Input: part model. Units: mm. Frame: model coordinates. A direction names the side the tool comes from. Coordinates: 2 decimals unless noted, no trailing zeros. Order: outer loops, then holes, each group sorted by start corner. A loop starts at its lowest first (then second) coordinate and runs counter-clockwise, first axis right, second up.
from build123d import *

# Parameters (mm, degrees)
MODEL_R                 = 6
MODEL_W                 = 3
MODEL_H                 = 24
SALIENTE_EXTRUIR2_DEPTH = 3


with BuildPart() as part:
    # Model → Saliente-Extruir2 (new body)
    with BuildSketch(Plane.XY):
        Polygon((-39.51128192, -9.185059482), (-32.41128192, -9.185059482), (-32.41128192, 2.614940518), (-9.21128192, 2.614940518), (-9.21128192, -9.185059482), (16.002025332, -9.185059482), (50.517196398, -9.185059482), (78.48871808, -9.185059482), (89.48871808, -9.185059482), (96.48871808, -9.185059482), (103.48871808, -9.185059482), (108.48871808, -9.185059482), (108.48871808, 88.814940518), (24.48871808, 88.814940518), (2.28871808, 88.814940518), (-0.51128192, 88.814940518), (-1.51128192, 88.814940518), (-9.21128192, 88.814940518), (-9.21128192, 77.014940518), (-32.41128192, 77.014940518), (-32.41128192, 88.814940518), (-39.51128192, 88.814940518), align=None)
        with Locations((-12.040844912, 39.714244751)):
            Circle(MODEL_R, mode=Mode.SUBTRACT)
        with Locations((-31.01128192, 39.814940518)):
            Rectangle(MODEL_W, MODEL_H, mode=Mode.SUBTRACT)
    extrude(amount=SALIENTE_EXTRUIR2_DEPTH)


solid = part.part
Item 1: Cut plane D-D on x = -28. Return loops of the section in (y, z), then the cut area to 3 significant figures.
Response values:
outline: (2.61, 0) - (77.01, 0) - (77.01, 3) - (2.61, 3) - close
area: 223 mm2
Item 2: Cut plane C-C on y = 42. Return loops of the section in (x, z).
Response values:
outline: (-39.51, 0) - (-32.51, 0) - (-32.51, 3) - (-39.51, 3) - close; (-29.51, 0) - (-17.59, 0) - (-17.59, 3) - (-29.51, 3) - close; (-6.49, 0) - (108.49, 0) - (108.49, 3) - (-6.49, 3) - close
Item 3: Ray query, probe 1 along Y at (x, z) = (-30, 0.2); probe 2 along X at (y, z) = (34.5, 0.75); probe 3 along X at (y, z) = (0, 0.3). Return the intervals inside material, ascending.
Response values:
probe 1: y = 2.61 to 27.81, 51.81 to 77.01
probe 2: x = -39.51 to -32.51, -29.51 to -15.01, -9.07 to 108.49
probe 3: x = -39.51 to -32.41, -9.21 to 108.49
Item 4: Pin query (flat end, axial travel): pin 1 Ø1.5 at (x, z) = (-31, 1) entering from +Y. Return the tip coordinate at first contact, or that it passes through.
Response values:
pin 1: stops at y = 77.01
Item 5: Access query for faces 4 (the face through (-31, 51.815, 1)), 5 (the face through (-32.411, 83, 1)), 6 (the face through (108.489, 39, 1)), 7 (the face through (33, 41, 3)), 8 (the face through (-32.411, -3, 1)). Directions: +Z, -Z, +X, -X, +Y, -Y. A direction counts if a zero-diameter tool reaches every point of the face in a straight line with its end or side. Return the directions, or none.
Response values:
face 4: +Z, -Z
face 5: +Z, -Z, +Y
face 6: +Z, -Z, +X, +Y, -Y
face 7: +Z, +X, -X, +Y, -Y
face 8: +Z, -Z, -Y
Item 6: Cut plane B-B on z = 2.1. Return loops of the section in (x, y), then the cut area to 3 significant figures.
Response values:
outline: (-39.51, -9.19) - (-32.41, -9.19) - (-32.41, 2.61) - (-9.21, 2.61) - (-9.21, -9.19) - (108.49, -9.19) - (108.49, 88.81) - (-9.21, 88.81) - (-9.21, 77.01) - (-32.41, 77.01) - (-32.41, 88.81) - (-39.51, 88.81) - close; hole (-32.51, 27.81) - (-29.51, 27.81) - (-29.51, 51.81) - (-32.51, 51.81) - close; hole circle Ø12 at (-12.04, 39.71)
area: 13,800 mm2
Item 7: Cut plane A-A on y = 29.5. Return loops of the section in (x, z), then the cut area to 3 significant figures.
Response values:
outline: (-39.51, 0) - (-32.51, 0) - (-32.51, 3) - (-39.51, 3) - close; (-29.51, 0) - (108.49, 0) - (108.49, 3) - (-29.51, 3) - close
area: 435 mm2
Item 8: Draft query along X for faces 1 (the face through (-31, 27.815, 1)), 2 (the face through (-39.511, 41, 1)), 3 (the face through (50, 88.815, 1)). Return one class per face: pulls with the +X half, pulls with the -X half, needs draft (parallel to the pull), parting line crosses it, or undercut.
Response values:
face 1: undercut
face 2: pulls with the -X half
face 3: needs draft
